Design review of the part built by this model. Coordinates are the model's own, in mm. A direction names the side the tool comes from. Give positions to 0.01 mm unless a question says otherwise; leave off trailing zeros. Order: outer loops, then holes, each group sorted by start corner. A loop starts at its lowest first (then second) coordinate and runs counter-clockwise, first axis right, second up. Notation, with made-up numbers: (66.5, 13) -> (90.5, 13) arc R31 ccw to (90.5, 43) -> close; hole circle Ø10 at (61, 82.25). An arc over 180 degrees is marked (long way). One line per item, written item: value. Start each with the question number.
1) Consider section D-D (y = 0.25). State the section outline as (x, z) points, plus the area to 3 significant figures.
2) Consider section C-C (z = 4.25). State the section outline as (x, y) points, plus the area to 3 significant figures.
3) Consider section B-B (x = 0). State the section outline as (y, z) points, plus the area to 3 significant figures.
4) Consider section A-A (y = 7.25). State the section outline as (x, z) points.
5) Tool access review of faces 1 (the face through (-9.611, -7, 5)), 2 (the face through (-20, 0, 10)), 3 (the face through (-9.611, 7, 5)): name each direction out of +Z, -Z, +X, -X, +Y, -Y from which nothing blocks a thin tool from reaching the whole face with its end or side.
6) Wall thickness on line 1 along Z through (x, y) = (-14, 3); line 2 along X through (y, z) = (8, 6.5); line 3 along X through (y, z) = (1.5, 3): over which ranges is each line inside the solid? List them lowest first. Write a range as from..to.
7) For pin 1 (6 mm diameter, centred on x = -24.5, y = -4.5, fed in from +Z); pin 2 (6 mm diameter, centred on x = -4, z = 9, fed in from +Y); pin 3 (4 mm diameter, centred on y = -6, z = 2.5, fed in from +X), all flat-tipped, find the tip position at first contact; note any pin that passes through.
from build123d import *

# Parameters (mm, degrees)
F0_W     = 20
F0_H     = 10
F1_DEPTH = 10
F2_DEPTH = 5


with BuildPart() as f1:
    # F0 (on Front) → F1 (new body)
    with BuildSketch(Plane.XZ):
        with BuildLine():
            ThreePointArc((-2.221403, 18.644934), (-1.860462, 14.492448), (2.285223, 14.924558))
            ThreePointArc((2.285223, 14.924558), (2.758486, 15.781217), (2.922367, 16.746093))
            ThreePointArc((2.922367, 16.746093), (1.012046, 19.487624), (-2.221403, 18.644934))
        make_face()
        with Locations((-19.611036, 5)):
            Rectangle(F0_W, F0_H)
    extrude(amount=F1_DEPTH)



with BuildPart() as f2:
    # F0 (on Front) → F2 (new body)
    with BuildSketch(Plane.XZ):
        with BuildLine():
            Line((-9.611036, 10), (-9.611036, 0))
            Line((-9.611036, 0), (2.285223, 14.924558))
            ThreePointArc((2.285223, 14.924558), (-1.860462, 14.492448), (-2.221403, 18.644934))
            Line((-2.221403, 18.644934), (-9.611036, 10))
        make_face()
    extrude(amount=F2_DEPTH)


with BuildPart() as f1_1:
    add(f1.part)

    add(f2.part)  # F3 merges F2
    # F3: F1 across plane


with BuildPart() as f1_2:
    add(f1_1.part)
    add(f1_1.part.mirror(Plane.XZ))


solid = f1_2.part
Checked values:
1. outline: (-29.61, 0) -> (-9.61, 0) -> (2.29, 14.92) arc R2.92 ccw to (2.92, 16.75) arc R2.92 ccw to (-2.22, 18.64) -> (-9.61, 10) -> (-29.61, 10) -> close
1. area: 306 mm^2
2. outline: (-29.61, -10) -> (-9.61, -10) -> (-9.61, -5) -> (-6.22, -5) -> (-6.22, 5) -> (-9.61, 5) -> (-9.61, 10) -> (-29.61, 10) -> close
2. area: 434 mm^2
3. outline: (-10, 13.82) -> (-5, 13.82) -> (-5, 12.06) -> (5, 12.06) -> (5, 13.82) -> (10, 13.82) -> (10, 19.67) -> (-10, 19.67) -> close
3. area: 135 mm^2
4. outline: (-29.61, 0) -> (-9.61, 0) -> (-9.61, 10) -> (-29.61, 10) -> close; (2.29, 14.92) arc R2.92 ccw to (2.92, 16.75) arc R2.92 ccw (long way) to start
5. face 1: +Z, -Z, +X, -Y
5. face 2: +Z, -X, +Y, -Y
5. face 3: +Z, -Z, +X, +Y
6. line 1: z = 0..10
6. line 2: x = -29.61..-9.61
6. line 3: x = -29.61..-7.22
7. pin 1: stops at z = 10
7. pin 2: stops at y = 5
7. pin 3: stops at x = -6.24
